Autodesk Inventor part; units mm, degrees
ref_plane "GUS_4502_1_XY" through (0, 0, 0) normal (1, 0, 0) x (0, 0, -1)
ref_plane "GUS_4502_1_YZ" through (0, 0, 0) normal (0, 0, -1) x (0, 1, 0)
ref_plane "GUS_4502_1_ZX" through (0, 0, 0) normal (0, 1, 0) x (1, 0, 0)
sketch "Skizze_1" plane through (0, 0, 0) normal (1, 0, 0) x (0, 1, 0)
  line L0 (-7, 7) -> (-7, -7)
  line L1 (-7, -7) -> (7, -7)
  line L2 (7, -7) -> (7, 7)
  line L3 (7, 7) -> (-7, 7)
  circle A0 centre (0, 0) radius 4.1
extrude "Extrusion1" add sketch "Skizze_1" along normal blind 5
sketch "Skizze_2" plane through (5, 0, 0) normal (1, 0, 0) x (0, 0, -1)
  line L0 (-7, 5) -> (-7, -5)
  line L1 (-7, -5) -> (-5, -5)
  line L2 (-5, -5) -> (-5, -7)
  line L3 (-5, -7) -> (5, -7)
  line L4 (5, -7) -> (5, -5)
  line L5 (5, -5) -> (7, -5)
  line L6 (7, -5) -> (7, 5)
  line L7 (7, 5) -> (5, 5)
  line L8 (5, 5) -> (5, 7)
  line L9 (5, 7) -> (-5, 7)
  line L10 (-5, 7) -> (-5, 5)
  line L11 (-5, 5) -> (-7, 5)
extrude "Extrusion2" cut sketch "Skizze_2" against normal blind 1
ref_plane "GUS_4502_1_XY" through (0, 0, 0) normal (1, 0, 0) x (0, 0, -1)
ref_plane "GUS_4502_1_YZ" through (0, 0, 0) normal (0, 0, -1) x (0, 1, 0)
ref_plane "GUS_4502_1_ZX" through (0, 0, 0) normal (0, 1, 0) x (1, 0, 0)
properties part number "Robotunits GUS_4502"
Verification items for the finished model (mm, model axes). A direction names the side the tool comes from. Give positions to 0.01 mm unless a question says otherwise; leave off trailing zeros. Write each loop counter-clockwise with the first axis right and the second up, starting at its lowest first coordinate (ties: lowest second). Pieces come first, ordered by that corner, then holes. Notation, with made-up numbers: M -14,36.5 L 15,36.5 A19 ccw 15,52.5 Z; hole C 41.25,-29.75 d11. An arc over 180 degrees is marked long. One line per question, with ' | ' between items.
1) Section check D-D on x = 0.95. Enter the section's corners in (y, z), plus the area to 3 significant figures.
Result:
outline: M -7,-7 L 7,-7 L 7,7 L -7,7 Z; hole C 0,0 d8.2 | area: 143 mm2
2) Section check A-A on x = 4.6. Enter the section's corners in (y, z).
Result:
outline: M -7,-7 L -5,-7 L -5,-5 L -7,-5 Z; M -7,5 L -5,5 L -5,7 L -7,7 Z; M 5,-7 L 7,-7 L 7,-5 L 5,-5 Z; M 5,5 L 7,5 L 7,7 L 5,7 Z
3) Thickness scan on line 1 along Y through (x, z) = (3.05, 0); line 2 along X through (y, z) = (-3.25, -4). Record the ranges inside material, lowest first. Write a range as [from, to].
Result:
line 1: y = [-7, -4.1], [4.1, 7] | line 2: x = [0, 4]
4) Section check B-B on z = 0. Enter the section's corners in (x, y).
Result:
outline: M 0,-7 L 4,-7 L 4,-4.1 L 0,-4.1 Z; M 0,4.1 L 4,4.1 L 4,7 L 0,7 Z
5) Mould release check, pull along Z, two halves, no side actions. Record for faces 4 (the flat face through (4.5, -6, 5)), 5 (the flat face through (4.5, -5, 6)), 6 (the flat face through (2, 0, -7)), 7 (the flat face through (2, 0, 7)): released by +Z, released by -Z, zero draft, split by the parting line, or undercut.
Result:
face 4: undercut | face 5: zero draft | face 6: released by -Z | face 7: released by +Z
6) Gauge pin test, flat ends, axial feed: pin 1 Ø4 at (y, z) = (-3, 0) entering from -X; pin 2 Ø4 at (y, z) = (3, 3.5) entering from +X. Record the tip position at first contact, or that the pin passes through.
Result:
pin 1: stops at x = 0 | pin 2: stops at x = 4
7) Set-up check for faces 1 (the flat face through (4.5, -6, -5)), 2 (the flat face through (2, 7, 0)), 3 (the flat face through (4.5, -5, -6)): record each of +Z, -Z, +X, -X, +Y, -Y from which the full face is reachable in a straight line by a thin tool's end or side.
Result:
face 1: +X, +Y, -Y | face 2: +Z, -Z, +X, -X, +Y | face 3: +Z, -Z, +X
